Input: part model. Units: mm. Frame: model coordinates. Give positions to 0.01 mm unless a question says otherwise; leave off trailing zeros. Loops run counter-clockwise (first coordinate to the right, second up) from the corner with the lowest first, then second, coordinate; pieces in that order, holes last. Notation, with made-up numbers: (73.25, 43) - (113.25, 43) arc R34 cw to (113.25, 73) - close; hole circle Ø1 at (54.5, 17). An arc over 180 degrees is marked (long way). Answer as a JSON object with one key per item and string values.
from build123d import *

# Parameters (mm, degrees)
RESSALTO_EXTRUS_O1_DEPTH        = 2
ESBO_O2_R                       = 1.5
CORTE_EXTRUS_O1_DEPTH           = 3
CORTE_EXTRUS_O1_TAPER           = -40
ESPELHAR3_COPY_1_SKETCH_R       = 1.5
ESPELHAR3_COPY_1_DEPTH          = 3
ESPELHAR3_COPY_1_TAPER          = -40
PADR_OCIRCULAR1_COUNT           = 2
PADR_OCIRCULAR1_ANGLE           = 90
PADR_OCIRCULAR1_COPY_1_SKETCH_R = 1.5
PADR_OCIRCULAR1_COPY_1_DEPTH    = 3
PADR_OCIRCULAR1_COPY_1_TAPER    = -40
PADR_OCIRCULAR1_COPY_2_SKETCH_R = 1.5
PADR_OCIRCULAR1_COPY_2_DEPTH    = 3
PADR_OCIRCULAR1_COPY_2_TAPER    = -40
PADR_OCIRCULAR1_COPY_3_SKETCH_R = 1.5
PADR_OCIRCULAR1_COPY_3_DEPTH    = 3
PADR_OCIRCULAR1_COPY_3_TAPER    = -40


with BuildPart() as part:
    # Esboço1 → Ressalto-extrusão1 (new body)
    with BuildSketch(Plane(origin=(0, 0, 0), x_dir=(1, 0, 0), z_dir=(0, 1, 0))):
        with BuildLine():
            Line((-20, 35), (-20, 45))
            Line((-20, 45), (0, 45))
            Line((0, 45), (0, 16))
            ThreePointArc((0, 16), (-16, 0), (0, -16))
            Line((0, -16), (0, -45))
            Line((0, -45), (-20, -45))
            Line((-20, -45), (-20, -35))
            Line((-20, -35), (-35, -20))
            Line((-35, -20), (-45, -20))
            Line((-45, -20), (-45, 20))
            Line((-45, 20), (-35, 20))
            Line((-35, 20), (-20, 35))
        make_face()
    ressalto_extrus_o1 = extrude(amount=RESSALTO_EXTRUS_O1_DEPTH)

    # Espelhar1: Ressalto-extrusão1 across plane
    add(ressalto_extrus_o1.mirror(Plane(origin=(0, 2, -16), x_dir=(0, 0, 1), z_dir=(-1, 0, 0))))

    # Esboço2 → Corte-extrusão1 (cut, through all)
    with BuildSketch(Plane(origin=(0, 2, 0), x_dir=(1, 0, 0), z_dir=(0, 1, 0))):
        with Locations((-15, 37)):
            Circle(ESBO_O2_R)
    corte_extrus_o1 = extrude(amount=-CORTE_EXTRUS_O1_DEPTH, taper=CORTE_EXTRUS_O1_TAPER, mode=Mode.SUBTRACT)

    # Espelhar2: Corte-extrusão1 across plane
    add(corte_extrus_o1.mirror(Plane(origin=(0, 0, 0), x_dir=(0, 0, 1), z_dir=(1, 0, 0))), mode=Mode.SUBTRACT)

    # Espelhar3: Corte-extrusão1 across plane
    add(corte_extrus_o1.mirror(Plane.XY), mode=Mode.SUBTRACT)

    # Espelhar3 copy 1 sketch → Espelhar3 copy 1 (cut, through all)
    with BuildSketch(Plane(origin=(0, 2, 0), x_dir=(-1, 0, 0), z_dir=(0, 1, 0))):
        with Locations((-15, 37)):
            Circle(ESPELHAR3_COPY_1_SKETCH_R)
    extrude(amount=-ESPELHAR3_COPY_1_DEPTH, taper=ESPELHAR3_COPY_1_TAPER, mode=Mode.SUBTRACT)

    # PadrãoCircular1: Corte-extrusão1 ×2 about axis
    padr_ocircular1_axis = Axis((0, 0, 0), (0, -1, 0))
    for i in range(1, PADR_OCIRCULAR1_COUNT):
        add(corte_extrus_o1.rotate(padr_ocircular1_axis, i * PADR_OCIRCULAR1_ANGLE / (PADR_OCIRCULAR1_COUNT - 1)), mode=Mode.SUBTRACT)

    # PadrãoCircular1 copy 1 sketch → PadrãoCircular1 copy 1 (cut, through all)
    with BuildSketch(Plane.ZX.offset(2)):
        with Locations((-15, -37)):
            Circle(PADR_OCIRCULAR1_COPY_1_SKETCH_R)
    extrude(amount=-PADR_OCIRCULAR1_COPY_1_DEPTH, taper=PADR_OCIRCULAR1_COPY_1_TAPER, mode=Mode.SUBTRACT)

    # PadrãoCircular1 copy 2 sketch → PadrãoCircular1 copy 2 (cut, through all)
    with BuildSketch(Plane(origin=(0, 2, 0), x_dir=(0, 0, -1), z_dir=(0, 1, 0))):
        with Locations((-15, 37)):
            Circle(PADR_OCIRCULAR1_COPY_2_SKETCH_R)
    extrude(amount=-PADR_OCIRCULAR1_COPY_2_DEPTH, taper=PADR_OCIRCULAR1_COPY_2_TAPER, mode=Mode.SUBTRACT)

    # PadrãoCircular1 copy 3 sketch → PadrãoCircular1 copy 3 (cut, through all)
    with BuildSketch(Plane(origin=(0, 2, 0), x_dir=(0, 0, -1), z_dir=(0, 1, 0))):
        with Locations((-15, -37)):
            Circle(PADR_OCIRCULAR1_COPY_3_SKETCH_R)
    extrude(amount=-PADR_OCIRCULAR1_COPY_3_DEPTH, taper=PADR_OCIRCULAR1_COPY_3_TAPER, mode=Mode.SUBTRACT)


solid = part.part
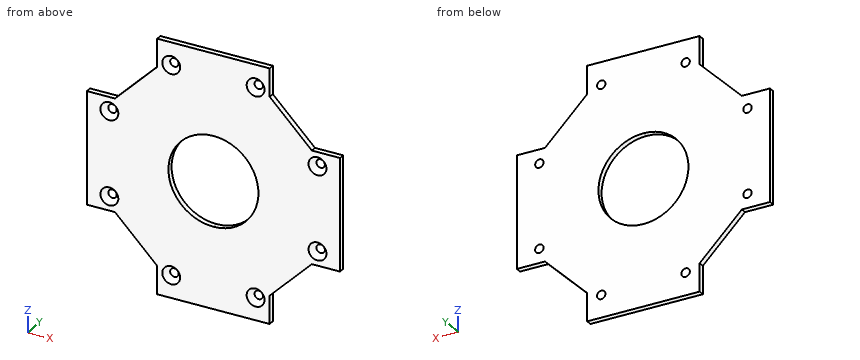
Item 1: Cut plane B-B (y = 0.4). Give the number of separate pieces and of enclosed holes in the cut face, then the cut area to 3 significant figures.
Geometry check:
{"separate pieces": "1", "enclosed holes": "9", "area": "5,040 mm2"}
Item 2: Cut plane A-A (z = 6). Return loops of the section in (x, y), then the cut area to 3 significant figures.
Geometry check:
{"outline": "(-45, 0) - (-14.83, 0) - (-14.83, 2) - (-45, 2) - close; (14.83, 0) - (45, 0) - (45, 2) - (14.83, 2) - close", "area": "121 mm2"}
Item 3: Material intervals for line 1 (Z direction, x = -36, y = 1.1); line 2 (Z direction, x = -38, y = 1.95); line 3 (X direction, y = 1.75, z = 3.5), sorted ascending. Write a range as [from, to].
Geometry check:
{"line 1": "z = [-20, -17.02], [-12.98, 12.98], [17.02, 20]", "line 2": "z = [-20, -16.17], [-13.83, 13.83], [16.17, 20]", "line 3": "x = [-45, -15.61], [15.61, 45]"}
Item 4: Contact query for flat-ended pins moving along their axis: P1, Ø1, axis at y = 1.5, z = 37.5, coming from the -X side; P2, Ø0.6, axis at y = 0.5, z = 40.5, coming from the +X side; P3, Ø0.6, axis at x = -40.5, y = 1, coming from the -Z side. Output: stop coordinate, or through.
Geometry check:
{"P1": "stops at x = -20", "P2": "stops at x = 20", "P3": "stops at z = -20"}
Item 5: Cut plane C-C (x = -5). Return loops of the section in (y, z).
Geometry check:
{"outline": "(0, -45) - (2, -45) - (2, -15.2) - (0, -15.2) - close; (0, 15.2) - (2, 15.2) - (2, 45) - (0, 45) - close"}
